from build123d import *

# Parameters (mm, degrees)
SKETCH_1_R          = 17
SKETCH_1_R_2        = 7
SKETCH_1_R_3        = 2
EXTRUDE_1_DEPTH     = 7
SKETCH_2_R          = 3
CUT_EXTRUDE_1_DEPTH = 3
CHAMFER_1_SIZE      = 1.5
CHAMFER_2_SIZE      = 0.5


with BuildPart() as part:
    # 草图1 → 凸台-拉伸1 (new body)
    with BuildSketch(Plane(origin=(0, 0, 0), x_dir=(0, 0, -1), z_dir=(1, 0, 0))):
        Circle(SKETCH_1_R)
        Circle(SKETCH_1_R_2, mode=Mode.SUBTRACT)
        with Locations((0, 12)):
            Circle(SKETCH_1_R_3, mode=Mode.SUBTRACT)
        with Locations((10.392304845, -6)):
            Circle(SKETCH_1_R_3, mode=Mode.SUBTRACT)
        with Locations((-10.392304845, -6)):
            Circle(SKETCH_1_R_3, mode=Mode.SUBTRACT)
    extrude(amount=EXTRUDE_1_DEPTH)

    # 草图2 → 切除-拉伸1 (cut)
    with BuildSketch(Plane(origin=(7, 0, 0), x_dir=(0, 0, -1), z_dir=(1, 0, 0))):
        with Locations((0, 12)):
            Circle(SKETCH_2_R)
        with Locations((10.392304845, -6)):
            Circle(SKETCH_2_R)
        with Locations((-10.392304845, -6)):
            Circle(SKETCH_2_R)
    extrude(amount=-CUT_EXTRUDE_1_DEPTH, mode=Mode.SUBTRACT)

    # 倒角1
    chamfer_1_edges = [part.edges().sort_by_distance(p)[0] for p in [
        (7, 0, 7),
    ]]
    chamfer(chamfer_1_edges, length=CHAMFER_1_SIZE)

    # 倒角2
    chamfer_2_edges = [part.edges().sort_by_distance(p)[0] for p in [
        (7, 0, 17),
    ]]
    chamfer(chamfer_2_edges, length=CHAMFER_2_SIZE)


solid = part.part
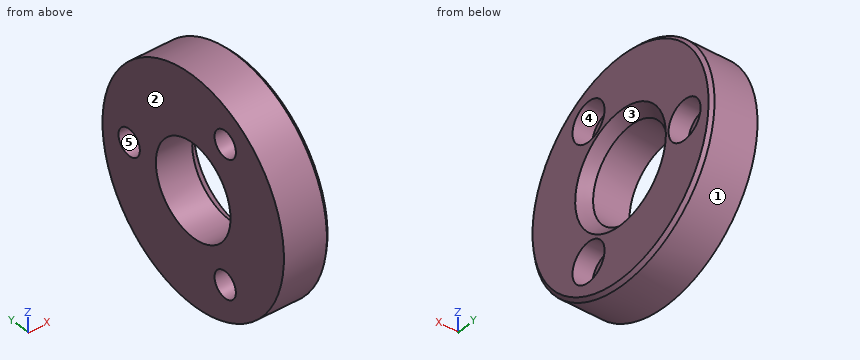
Read the model definition and answer for the solid it produces. Units are mm, in the model's axes. Face numbers are marked on the shaded views. A direction names the side the tool comes from. Coordinates: 2 decimals unless noted, no trailing zeros. Write each loop counter-clockwise with the first axis right and the second up, starting at its lowest first coordinate (ties: lowest second). Pieces come first, ordered by that corner, then holes. Notation, with made-up numbers: M 83,12 L 126,12 A18 ccw 126,29 Z; hole C -18.75,-20.75 d7. An arc over 180 degrees is marked long. Use a Markdown table: item, result.
Q1. The part is cut by section B-B, the plane x = 2.75. Write down the section's boundary in (y, z), then the cut area to 3 significant figures.
Answer block:
| item | result |
|---|---|
| outline | C 0,0 d34; hole C -6,-10.39 d4; hole C -6,10.39 d4; hole C 0,0 d14; hole C 12,0 d4 |
| area | 716 mm2 |
Q2. Determine the mould class of the marked faces 1, 2 and 3 for opening direction Y: released by +Y, released by -Y, zero draft, split by the parting line, or undercut.
Answer block:
| item | result |
|---|---|
| face 1 | split by the parting line |
| face 2 | zero draft |
| face 3 | undercut |
Q3. The part is cut by section A-A, the plane z = 0. Write down the section's boundary in (x, y), then the cut area to 4 significant figures.
Answer block:
| item | result |
|---|---|
| outline | M 0,-17 L 6.5,-17 L 7,-16.5 L 7,-8.5 L 5.5,-7 L 0,-7 Z; M 0,7 L 5.5,7 L 7,8.5 L 7,9 L 4,9 L 4,10 L 0,10 Z; M 0,14 L 4,14 L 4,15 L 7,15 L 7,16.5 L 6.5,17 L 0,17 Z |
| area | 103.5 mm2 |
Q4. The part is cut by section C-C, the plane y = -6. Give the number of separate pieces and of enclosed holes in the cut face, then the cut area to 3 significant figures.
Answer block:
| item | result |
|---|---|
| separate pieces | 4 |
| enclosed holes | 0 |
| area | 100 mm2 |
Q5. Straight lines are drawn through the part: L1, parallel to Y at x = 3.2, z = 0; L2, parallel to Z at x = 6, y = -5; L3, parallel to Y at x = 4.25, z = 0. For each, find the intervals that lie inside material, in ascending order. Write a range as [from, to].
Answer block:
| item | result |
|---|---|
| L1 | y = [-17, -7], [7, 10], [14, 17] |
| L2 | z = [-16.25, -13.22], [-7.56, -5.59], [5.59, 7.56], [13.22, 16.25] |
| L3 | y = [-17, -7], [7, 9], [15, 17] |
Q6. Each of these flat-tipped pins is pushed along its axis until it touches: pin 1 Ø3 at (x, y) = (1, -7.5) entering from -Z; pin 2 Ø2.5 at (y, z) = (-6, -10.39) entering from +X; pin 3 Ø4 at (x, z) = (5.5, -2.5) entering from +Y; pin 4 Ø1.5 at (x, z) = (6, -8) entering from -Y. Where does it stop, or does it pass through?
Answer block:
| item | result |
|---|---|
| pin 1 | stops at z = -15.91 |
| pin 2 | passes through |
| pin 3 | stops at y = 16.99 |
| pin 4 | stops at y = -15.38 |
Q7. Which of the six approach directions +Z, -Z, +X, -X, +Y, -Y give full straight-line access (tool end or side, diameter ignored) to the marked faces 4 and 5?
Answer block:
| item | result |
|---|---|
| face 4 | +X |
| face 5 | +X, -X |
